from build123d import *

# Parameters (mm, degrees)
SK_BRACKET_FACE_W  = 3
SK_BRACKET_FACE_H  = 44.5
BRACKET_FACE_DEPTH = 22.5
SK_BRACKET_TOP_W   = 33
SK_BRACKET_TOP_H   = 3
BRACKET_TOP_DEPTH  = 22.5


with BuildPart() as part:
    # SK_Gearmotor → Gearmotor (revolve)
    with BuildSketch(Plane(origin=(0, 0, 0), x_dir=(1, 0, 0), z_dir=(0, 1, 0)), mode=Mode.PRIVATE) as gearmotor_sk:
        Polygon((0, 18), (3, 18), (3, 0), (18.5, 0), (18.5, -70), (0, -70), align=None)
    revolve(gearmotor_sk.sketch.rotate(Axis((0, 0, -23), (0, 0, 1)), 180), axis=Axis((0, 0, -23), (0, 0, 1)))

    # SK_Bracket_Face → Bracket_Face (add, symmetric)
    with BuildSketch(Plane(origin=(0, 0, 0), x_dir=(0, 0, -1), z_dir=(1, 0, 0))):
        with Locations((1.5, -0.25)):
            Rectangle(SK_BRACKET_FACE_W, SK_BRACKET_FACE_H)
    extrude(amount=BRACKET_FACE_DEPTH, both=True)

    # SK_Bracket_Top → Bracket_Top (add, symmetric)
    with BuildSketch(Plane(origin=(0, 0, 0), x_dir=(0, 0, -1), z_dir=(1, 0, 0))):
        with Locations((-13.5, 20.5)):
            Rectangle(SK_BRACKET_TOP_W, SK_BRACKET_TOP_H)
    extrude(amount=BRACKET_TOP_DEPTH, both=True)


solid = part.part
CAD build for the part. Positions are in the model's coordinates, mm. A direction names the side the tool comes from. Coordinates: 2 decimals unless noted, no trailing zeros. Loops run counter-clockwise (first coordinate to the right, second up) from the corner with the lowest first, then second, coordinate; pieces in that order, holes last. Notation, with made-up numbers: (-21, 32.5) - (22, 32.5) arc R13 ccw to (22, 42.5) - close; hole circle Ø11 at (11.5, -11). An arc over 180 degrees is marked (long way). Use one line per item in the form item = value. Start each with the question number.
1) Band-saw the part on C-C (y = 0). Give the cut face in (x, z), and give its area (4 significant figures).
2) Band-saw the part on A-A (z = 17.5). Give the cut face in (x, y), and give its area (3 significant figures).
3) Band-saw the part on B-B (x = 0). Give the cut face in (y, z), and give its area (3 significant figures).
4) Flat gauge pins, fed straight in: pin 1 (2 mm diameter, centred on y = 16, z = 37.5, fed in from +X); pin 2 (1.5 mm diameter, centred on y = 3, z = 31.5, fed in from -X); pin 3 (24 mm diameter, centred on x = -8.5, z = 15.5, fed in from -Y). Where does each tip first touch, or does it go through?
5) Band-saw the part on D-D (z = 62). Give the cut face in (x, y).
6) Two-plate mould, pull along Y, no slides. Class faces 4 (the face through (0, 22, 14)), 5 (the face through (10, -16, 0)), 6 (the face through (0, 0, -18)): +Y half, -Y half, draft (parallel to the pull), parting line (faces both ways), or undercut.
7) Drill centre lines: L1, parallel to Z at x = -9, y = 0.5; L2, parallel to Z at x = 20.5, y = -17; L3, parallel to Y at x = -2, z = 2. Where is each one in solid material? Low to high. Write a range as from..to.
8) Tool access for faces 1 (the face through (0, 19, 15)), 2 (the face through (-2.86, -0.9, -10.4)), 3 (the face through (0, 20, 30)): list every direction of +Z, -Z, +X, -X, +Y, -Y with a clear straight run to the whole face (end or side of a thin tool).
Check values:
q1.outline = (-22.5, -3) - (-3, -3) - (-3, -18) - (3, -18) - (3, -3) - (22.5, -3) - (22.5, 0) - (18.5, 0) - (18.5, 70) - (-18.5, 70) - (-18.5, 0) - (-22.5, 0) - close
q1.area = 2,815 mm2
q2.outline = (-22.5, 19) - (22.5, 19) - (22.5, 22) - (-22.5, 22) - close; circle Ø37 at (0, 0)
q2.area = 1,210 mm2
q3.outline = (-22.5, -3) - (-3, -3) - (-3, -18) - (3, -18) - (3, -3) - (22, -3) - (22, 30) - (19, 30) - (19, 0) - (18.5, 0) - (18.5, 70) - (-18.5, 70) - (-18.5, 0) - (-22.5, 0) - close
q3.area = 2,900 mm2
q4.pin_1 = 10.83
q4.pin_2 = -18.36
q4.pin_3 = -18.5
q5.outline = circle Ø37 at (0, 0)
q6.face_4 = +Y half
q6.face_5 = undercut
q6.face_6 = draft
q7.L1 = -3..70
q7.L2 = -3..0
q7.L3 = -18.39..18.39, 19..22
q8.face_1 = +Z, +X, -X
q8.face_2 = -Z
q8.face_3 = +Z, +X, -X, +Y
